Could you check a few things on this model? Use its own coordinates, in mm. A direction names the side the tool comes from. Give positions to 0.01 mm unless a question says otherwise; leave off trailing zeros. Order: outer loops, then holes, each group sorted by start corner. A loop starts at its lowest first (then second) coordinate and runs counter-clockwise, first axis right, second up.
(1) Imagine slicing it at C-C, the plane z = 14. Write out the boundary of the cut face in (x, y) (3 decimals), then the cut area to 3 significant figures.
(2) Will these pins go through, and if not, where does the flat tip stop? pin 1 (0.8 mm diameter, centred on x = 0, z = 21.5, fed in from +Y) (3 decimals); pin 2 (1 mm diameter, centred on y = 0, z = 21.5, fed in from -X) (3 decimals); pin 3 (1 mm diameter, centred on x = 0, z = 20.5, fed in from -Y) (3 decimals); pin 4 (1 mm diameter, centred on x = 0, y = -0.5, fed in from -Z).
(3) If I drill on probe 1 along Z at (x, y) = (-0.3, 0.8); probe 2 along Y at (x, z) = (-0.4, -20) (3 decimals); probe 3 along X at (y, z) = (0.1, 7), over which ranges is the centre line in solid material (lowest first)?
(4) Imagine slicing it at A-A, the plane x = 0. Write out the boundary of the cut face in (y, z) (3 decimals).
(5) On a 3-axis mill with a long thin cutter (end or side, diameter ignored), from which of +Z, -Z, +X, -X, +Y, -Y can I reach the whole of each face in a straight line? I mean faces 1 (the flat face through (0, -0.475, 21)), 2 (the flat face through (0, 0.475, 21)), 3 (the flat face through (-0.475, 0, 21)). Say none if no direction works.
from build123d import *

# Parameters (mm, degrees)
SKETCH1_R           = 0.975
BOSS_EXTRUDE2_DEPTH = 18.75
SKETCH2_W           = 0.95
SKETCH2_H           = 0.95
BOSS_EXTRUDE3_DEPTH = 5


with BuildPart() as part:
    # Sketch1 → Boss-Extrude2 (new body)
    with BuildSketch(Plane.XY):
        Circle(SKETCH1_R)
    boss_extrude2 = extrude(amount=BOSS_EXTRUDE2_DEPTH)

    # Sketch2 → Boss-Extrude3 (add)
    with BuildSketch(Plane.XY.offset(18.75)):
        Rectangle(SKETCH2_W, SKETCH2_H)
    boss_extrude3 = extrude(amount=BOSS_EXTRUDE3_DEPTH)

    # Mirror1: Boss-Extrude2, Boss-Extrude3 across plane
    add(boss_extrude2.mirror(Plane.XY))
    add(boss_extrude3.mirror(Plane.XY))


solid = part.part
Answer block:
1. outline: circle Ø1.95 at (0, 0)
1. area: 2.99 mm2
2. pin 1: stops at y = 0.475
2. pin 2: stops at x = -0.475
2. pin 3: stops at y = -0.475
2. pin 4: stops at z = -23.75
3. probe 1: z = -18.75 to 18.75
3. probe 2: y = -0.475 to 0.475
3. probe 3: x = -0.97 to 0.97
4. outline: (-0.975, -18.75) - (-0.475, -18.75) - (-0.475, -23.75) - (0.475, -23.75) - (0.475, -18.75) - (0.975, -18.75) - (0.975, 18.75) - (0.475, 18.75) - (0.475, 23.75) - (-0.475, 23.75) - (-0.475, 18.75) - (-0.975, 18.75) - close
5. face 1: +Z, +X, -X, -Y
5. face 2: +Z, +X, -X, +Y
5. face 3: +Z, -X, +Y, -Y
